Check sheet for the modelled part. Datum: model origin and axes. Units: mm. A direction names the side the tool comes from. Round coordinates to 2 decimals unless told otherwise and drop trailing zeros. Order: outer loops, then holes, each group sorted by start corner. A loop starts at its lowest first (then second) coordinate and runs counter-clockwise, first axis right, second up.
Q1. Cross-section at B-B on z = 8.25. Record the cut outline in (x, y), then the cut area to 3 significant figures.
Q2. Depth check by flat-ended pin: P1, Ø2, axis at y = -1.5, z = 6, coming from the +X side; P2, Ø1, axis at y = 2, z = 1, coming from the -X side; P3, Ø2, axis at y = -5, z = 3, coming from the -X side. Enter the tip coordinate at first touch or a pass-through.
Q3. Set-up check for faces 1 (the cylindrical face through (6.214, 1.38, 7.74)), 2 (the flat face through (0, -6.365, 3)): record each of +Z, -Z, +X, -X, +Y, -Y from which the full face is reachable in a straight line by a thin tool's end or side.
Q4. Scan lines: probe 1 along X at (y, z) = (0, 8.1); probe 2 along Y at (x, z) = (0, 7.4); probe 3 along Y at (x, z) = (-4.75, 4.75). Record each from-to range of solid material in increasing order.
Solid Edge part; units mm, degrees
sketch "Sketch1" plane through (0, 0, 0) normal (0, 0, 1) x (1, 0, 0)
  line L0 (-3.675, 6.3653) -> (3.675, 6.3653)
  line L1 (3.675, 6.3653) -> (7.35, 0)
  line L2 (7.35, 0) -> (3.675, -6.3653)
  line L3 (3.675, -6.3653) -> (-3.675, -6.3653)
  line L4 (-3.675, -6.3653) -> (-7.35, 0)
  line L5 (-7.35, 0) -> (-3.675, 6.3653)
extrude "Protrusion1" add sketch "Sketch1" along normal blind 7
sketch "Sketch2" plane through (0, -5.5125, 6.3) normal (-1, 0, 0) x (0, 1, 0)
  line L0 (-2.267, 4.8858) -> (0.5614, 7.7142)
  line L1 (-2.267, 4.8858) -> (-2.267, 0.7142)
  line L2 (-2.267, 0.7142) -> (0.5614, -2.1142)
revolve "RevolvedCutout1" cut sketch "Sketch2" angle 360 about axis through (0, 0, 0.5943) along (0, 0, -1) material side at (0, -6.4007, -0.0354)
sketch "Sketch3" plane through (0, 0, 0) normal (1, 0, 0) x (0, 1, 0)
  line L0 (0, 9.5) -> (-5.3653, 9.5)
  arc A0 (-6.3653, 8.5) -> (-5.3653, 9.5) centre (-5.3653, 8.5) cw
  line L1 (-6.3653, 8.5) -> (-6.3653, 7)
  line L2 (-6.3653, 7) -> (0, 7)
  line L3 (0, 7) -> (0, 9.5)
revolve "RevolvedProtrusion1" add sketch "Sketch3" angle 360 about axis through (0, 0, -57) along (0, 0, 1)
hole "Hole_1" at (0, 0, 7) direction (0, 0, 1) diameter 6.647 end up to next both ways yes
sketch "Sketch4" plane through (0, 0, 9.5) normal (0, 0, 1) x (0, 1, 0)
  circle A0 centre (0, 0) radius 4.5
extrude "ExtrudedCutout_2" cut sketch "Sketch4" against normal blind 2
sketch "Sketch5" plane through (0, 0, 7.5) normal (0, 0, 1) x (0, 1, 0)
  circle A0 centre (0, 0) radius 4.5
  circle A1 centre (0, 0) radius 3.25
extrude "Protrusion2" add sketch "Sketch5" along normal up to vertex (2 mm away)
Results found:
1. outline: circle Ø12.73 at (0, 0); hole circle Ø6.5 at (0, 0)
1. area: 94.1 mm2
2. P1: stops at x = 7.06
2. P2: stops at x = -6.48
2. P3: stops at x = -5.04
3. face 1: +Z
3. face 2: +Z, -Z, +X, -X, -Y
4. probe 1: x = -6.37 to -3.25, 3.25 to 6.37
4. probe 2: y = -6.37 to -3.32, 3.32 to 6.37
4. probe 3: y = -4.5 to 4.5
